from build123d import *

# Parameters (mm, degrees)
F1_R      = 31.75
F2_DEPTH  = 279.4
F3_R      = 50.8
F4_DEPTH  = 50.8
F5_R      = 40.64
F6_DEPTH  = 12.7
F4_FACE_R = 50.8
F7_DEPTH  = 25.4
F8_W      = 27.653224
F8_H      = 75.585485
F9_DEPTH  = 7.62
F10_R     = 25.4
F11_DEPTH = 25.4
F12_R     = 8.89
F13_DEPTH = 5.08


with BuildPart() as f2:
    # F1 (on face) → F2 (new body)
    with BuildSketch(Plane.XY):
        with Locations((-63.058764, 27.092882)):
            Circle(F1_R)
    extrude(amount=-F2_DEPTH)

    # F3 (on face) → F4 (join)
    with BuildSketch(Plane(origin=(0, 0, -279.4), x_dir=(1, 0, 0), z_dir=(0, 0, -1))):
        with Locations((-63.058764, -27.092882)):
            Circle(F3_R)
    extrude(amount=F4_DEPTH)

    # F5 (on face) → F6 (join)
    with BuildSketch(Plane.XY):
        with Locations((-63.058764, 27.092882)):
            Circle(F5_R)
    extrude(amount=F6_DEPTH)

    # F4_face (on face) → F7 (cut)
    with BuildSketch(Plane(origin=(-63.058764, 27.092882, -330.2), x_dir=(1, 0, 0), z_dir=(0, 0, -1))):
        Circle(F4_FACE_R)
    extrude(amount=-F7_DEPTH, mode=Mode.SUBTRACT)

    # F8 (on Front) → F9 (join)
    with BuildSketch(Plane.XZ):
        with Locations((-63.074544, -166.380242)):
            Rectangle(F8_W, F8_H)
    extrude(amount=F9_DEPTH)

    # F10 (on face) → F11 (cut)
    with BuildSketch(Plane(origin=(0, 0, -304.8), x_dir=(1, 0, 0), z_dir=(0, 0, -1))):
        with Locations((-63.058764, -27.092882)):
            Circle(F10_R)
    extrude(amount=-F11_DEPTH, mode=Mode.SUBTRACT)

    # F12 (on face) → F13 (join)
    with BuildSketch(Plane.XZ.offset(7.62)):
        with Locations((-63.074544, -166.380242)):
            Circle(F12_R)
    extrude(amount=F13_DEPTH)


solid = f2.part
The model under review builds one solid part; all positions refer to its coordinate system, in mm. A direction names the side the tool comes from. Round coordinates to 2 decimals unless told otherwise and drop trailing zeros. Loops run counter-clockwise (first coordinate to the right, second up) from the corner with the lowest first, then second, coordinate; pieces in that order, holes last. Notation, with made-up numbers: M 71.25,7.25 L 77.25,7.25 A23 ccw 77.25,42.25 Z; hole C 52.5,77.25 d8. An arc over 180 degrees is marked long. Answer as CSV lines item,"result".
1. We need section A-A (y = 10). Give the boundary of the cut face in (x, z) (3 decimals), plus the area to 3 significant figures.
Outcome:
outline,"M -110.897,-304.8 L -81.847,-304.8 L -81.847,-279.4 L -44.271,-279.4 L -44.271,-304.8 L -15.221,-304.8 L -15.221,-279.4 L -36.303,-279.4 L -36.303,0 L -26.188,0 L -26.188,12.7 L -99.929,12.7 L -99.929,0 L -89.815,0 L -89.815,-279.4 L -110.897,-279.4 Z"
area,"17,400 mm2"
2. Draft analysis for pull direction Z (two halves, no side actions). For faces 4 (the face through (-64.232, -10.124, -157.566)), 5 (the face through (-66.37, 1.91, -292.28)), 6 (the face through (-63, 27, -279.4)), state which applies: pulls with the +Z half, pulls with the -Z half, needs draft (parallel to the pull), parting line crosses it, or undercut.
Outcome:
face 4,"undercut"
face 5,"needs draft"
face 6,"pulls with the -Z half"
3. For faces 1 (the face through (-95.309, 2.364, 6.261)), 2 (the face through (-63, -12.7, -166)), 3 (the face through (-45.99, 53.865, -137.744)), list the 3-axis set-ups (+Z, -Z, +X, -X, +Y, -Y) from which the entire face can be reached by the end or side of a thin tool; tool diameter is ignored.
Outcome:
face 1,"+Z"
face 2,"+X, -X, -Y"
face 3,"none"
4. To check wall thickness, follow L1, parallel to Z at x = -98, y = 14.5; L2, parallel to Z at x = -19.5, y = 9; L3, parallel to X at y = 8, z = -97. State the ranges of each line that lie inside material, in increasing order. Write a range as [from, to].
Outcome:
L1,"z = [-304.8, -279.4], [0, 12.7]"
L2,"z = [-304.8, -279.4]"
L3,"x = [-88.43, -37.69]"
5. We need section D-D (z = -109). Give the boundary of the cut face in (x, y), plus the area to 3 significant figures.
Outcome:
outline,"C -63.06,27.09 d63.5"
area,"3,170 mm2"
6. We need section B-B (z = -149.5). Give the boundary of the cut face in (x, y), plus the area to 3 significant figures.
Outcome:
outline,"M -76.9,-7.62 L -49.25,-7.62 L -49.25,-1.5 A31.75 ccw long -76.9,-1.48 Z"
area,"3,280 mm2"
7. We need section C-C (x = -42.5). Give the boundary of the cut face in (y, z), plus the area to 3 significant figures.
Outcome:
outline,"M -19.36,-304.8 L 12.18,-304.8 L 12.18,-279.4 L 42.01,-279.4 L 42.01,-304.8 L 73.55,-304.8 L 73.55,-279.4 L 51.29,-279.4 L 51.29,0 L 62.15,0 L 62.15,12.7 L -7.96,12.7 L -7.96,0 L 2.9,0 L 2.9,-279.4 L -19.36,-279.4 Z"
area,"16,000 mm2"
8. Insertion check: pin 1 Ø1 at (x, z) = (-33.5, -64) entering from -Y; pin 2 Ø6 at (y, z) = (47.5, -26.5) entering from +X; pin 3 Ø24.5 at (x, y) = (-53.5, 28) entering from -Z. Each pin has a flat end and moves straight along its axis. Give the tip position at first contact, or say it passes through.
Outcome:
pin 1,"stops at y = 14.3"
pin 2,"stops at x = -36.51"
pin 3,"stops at z = -279.4"
